Read the model definition and answer for the solid it produces. Units are mm, in the model's axes. Coordinates: 2 decimals unless noted, no trailing zeros. Write each loop counter-clockwise with the first axis right and the second up, starting at its lowest first coordinate (ties: lowest second). Pieces come first, ordered by that corner, then holes. Notation, with made-up numbers: (43.5, 32) -> (87.5, 32) arc R22 ccw to (87.5, 46) -> close; hole circle Ø2 at (-25, 50.5). An arc over 180 degrees is marked (long way). Use CSV: the item, a comma, the result in double quotes.
from build123d import *

# Parameters (mm, degrees)
SKETCH1_W           = 130
SKETCH1_H           = 430
BOSS_EXTRUDE1_DEPTH = 3
SKETCH2_W           = 30
SKETCH2_H           = 40
CUT_EXTRUDE1_DEPTH  = 10
SKETCH3_R           = 1.5
SKETCH3_R_2         = 1.6
SKETCH3_R_3         = 2.1
CUT_EXTRUDE2_DEPTH  = 10
SKETCH4_R           = 7
CUT_EXTRUDE3_DEPTH  = 10


with BuildPart() as part:
    # Sketch1 → Boss-Extrude1 (new body)
    with BuildSketch(Plane(origin=(0, 0, 0), x_dir=(1, 0, 0), z_dir=(0, 1, 0))):
        Rectangle(SKETCH1_W, SKETCH1_H)
    extrude(amount=BOSS_EXTRUDE1_DEPTH)

    # Sketch2 → Cut-Extrude1 (cut)
    with BuildSketch(Plane(origin=(0, 3, 0), x_dir=(1, 0, 0), z_dir=(0, 1, 0))):
        with Locations((0, -195)):
            Rectangle(SKETCH2_W, SKETCH2_H)
    extrude(amount=-CUT_EXTRUDE1_DEPTH, mode=Mode.SUBTRACT)

    # Sketch3 → Cut-Extrude2 (cut)
    with BuildSketch(Plane.XZ):
        with Locations(Location((-53.05, -3.75, 0), (0, 0, 270))):
            Circle(SKETCH3_R)
        with Locations(Location((-24.95, -3.75, 0), (0, 0, 270))):
            Circle(SKETCH3_R)
        with Locations(Location((-53.05, -106.75, 0), (0, 0, 270))):
            Circle(SKETCH3_R_2)
        with Locations(Location((-24.95, -106.75, 0), (0, 0, 270))):
            Circle(SKETCH3_R)
        with Locations(Location((24.95, -106.75, 0), (0, 0, 90))):
            Circle(SKETCH3_R)
        with Locations(Location((57.5, 202.5, 0), (0, 0, 270))):
            Circle(SKETCH3_R_3)
        with Locations(Location((53.05, -106.75, 0), (0, 0, 90))):
            Circle(SKETCH3_R_2)
        with Locations(Location((24.95, -3.75, 0), (0, 0, 90))):
            Circle(SKETCH3_R)
        with Locations(Location((-57.5, 202.5, 0), (0, 0, 270))):
            Circle(SKETCH3_R_3)
        with Locations(Location((53.05, -3.75, 0), (0, 0, 90))):
            Circle(SKETCH3_R)
        with Locations(Location((-41.5, 175, 0), (0, 0, 270))):
            Circle(SKETCH3_R_3)
        with Locations(Location((41.5, 175, 0), (0, 0, 270))):
            Circle(SKETCH3_R_3)
        with Locations(Location((41.5, -175, 0), (0, 0, 270))):
            Circle(SKETCH3_R_3)
        with Locations(Location((-41.5, -175, 0), (0, 0, 270))):
            Circle(SKETCH3_R_3)
    extrude(amount=-CUT_EXTRUDE2_DEPTH, mode=Mode.SUBTRACT)

    # Sketch4 → Cut-Extrude3 (cut)
    with BuildSketch(Plane.XZ):
        with Locations(Location((-17.5, 100.952208061, 0), (0, 0, 270))):
            Circle(SKETCH4_R)
        with Locations(Location((17.5, 100.952208061, 0), (0, 0, 270))):
            Circle(SKETCH4_R)
    extrude(amount=-CUT_EXTRUDE3_DEPTH, mode=Mode.SUBTRACT)


solid = part.part
1. A cutting plane is placed at B-B (x = -6). Give the vertices of the cut face in (y, z), and give its area (3 significant figures).
Solutions:
outline,"(0, -215) -> (3, -215) -> (3, 175) -> (0, 175) -> close"
area,"1,170 mm^2"
2. Find the intervals of material crossed by line 1 along X through (y, z) = (1.6, -3.75); line 2 along X through (y, z) = (1.1, -106.75); line 3 along Z through (x, y) = (24.95, 2.15), in increasing order.
Solutions:
line 1,"x = -65 to -54.55, -51.55 to -26.45, -23.45 to 23.45, 26.45 to 51.55, 54.55 to 65"
line 2,"x = -65 to -54.65, -51.45 to -26.45, -23.45 to 23.45, 26.45 to 51.45, 54.65 to 65"
line 3,"z = -215 to -108.25, -105.25 to -5.25, -2.25 to 215"
3. A cutting plane is placed at A-A (y = 2.1). Give the number of separate pieces and of enclosed holes in the cut face, and give its area (3 significant figures).
Solutions:
separate pieces,"1"
enclosed holes,"16"
area,"54,300 mm^2"
4. For a pull along X with two mould halves and no side action, classify faces 1 (the cylindrical face through (-20.181, 1.479, 94.486)), 2 (the flat face through (-1, 0, -3)) as pulls with the +X half, pulls with the -X half, needs draft (parallel to the pull), parting line crosses it, or undercut.
Solutions:
face 1,"undercut"
face 2,"needs draft"
5. This flat-tipped pin is pushed along its axis until it touches: pin 1 Ø1.8 at (x, z) = (-24.95, -3.75) entering from +Y. Where does it stop, or does it pass through?
Solutions:
pin 1,"passes through"
